CAD build for the part. Positions are in the model's coordinates, mm. Face numbers are marked on the shaded views. A direction names the side the tool comes from. Round coordinates to 2 decimals unless told otherwise and drop trailing zeros. Loops run counter-clockwise (first coordinate to the right, second up) from the corner with the lowest first, then second, coordinate; pieces in that order, holes last. Notation, with made-up numbers: M 25,63 L 84,63 A13 ccw 84,72 Z; hole C 56,32 d2. An arc over 180 degrees is marked long. Use a Markdown table: item, result. Add a question column.
(1) Band-saw the part on B-B, the plane z = 7.75. Give the number of separate pieces and of enclosed holes in the cut face, and give its area (3 significant figures).
(2) Wall check: L1, parallel to Z at x = 12.5, y = -11.5. Give the ranges that are in metal, low to high.
(3) Which spindle directions (+Z, -Z, +X, -X, +Y, -Y) get a long thin tool onto all of the face, cutting with end or side? Do the marked faces 1, 2 and 3. Say none if no direction does.
(4) Band-saw the part on C-C, the plane y = 3. Write the cut outline in (x, z).
(5) Band-saw the part on A-A, the plane y = -16. Write the cut outline in (x, z).
(6) Flat gauge pins, fed straight in: P1, Ø5, axis at x = -7.5, z = 8.5, coming from the +Y side; P2, Ø0.5, axis at y = -15, z = 5, coming from the -X side; P3, Ø3, axis at x = -5, z = 9, coming from the -Y side. Where does each tip first touch, or does it go through?
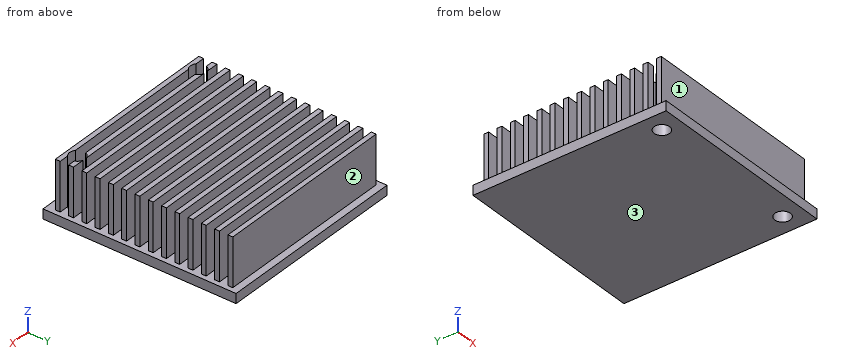
from build123d import *

# Parameters (mm, degrees)
SKETCH1_W           = 40
SKETCH1_H           = 40
BOSS_EXTRUDE1_DEPTH = 2
SKETCH2_W           = 38
SKETCH2_H           = 1
BOSS_EXTRUDE2_DEPTH = 10
SKETCH3_R           = 1.6
CUT_EXTRUDE1_DEPTH  = 13


with BuildPart() as part:
    # Sketch1 → Boss-Extrude1 (new body)
    with BuildSketch(Plane.XY):
        Rectangle(SKETCH1_W, SKETCH1_H)
    extrude(amount=BOSS_EXTRUDE1_DEPTH)

    # Sketch2 → Boss-Extrude2 (add)
    with BuildSketch(Plane.XY.offset(2)):
        with Locations((0, 15.280666702)):
            Rectangle(SKETCH2_W, SKETCH2_H)
        with Locations((0, 18.030666702)):
            Rectangle(SKETCH2_W, SKETCH2_H)
        with Locations((0, 12.530666702)):
            Rectangle(SKETCH2_W, SKETCH2_H)
        with Locations((0, 9.780666702)):
            Rectangle(SKETCH2_W, SKETCH2_H)
        with Locations((0, 7.030666702)):
            Rectangle(SKETCH2_W, SKETCH2_H)
        with Locations((0, 4.280666702)):
            Rectangle(SKETCH2_W, SKETCH2_H)
        with Locations((0, 1.530666702)):
            Rectangle(SKETCH2_W, SKETCH2_H)
        with Locations((0, -1.219333298)):
            Rectangle(SKETCH2_W, SKETCH2_H)
        with Locations((0, -3.969333298)):
            Rectangle(SKETCH2_W, SKETCH2_H)
        with Locations((0, -6.719333298)):
            Rectangle(SKETCH2_W, SKETCH2_H)
        with Locations((0, -9.469333298)):
            Rectangle(SKETCH2_W, SKETCH2_H)
        with Locations((0, -12.219333298)):
            Rectangle(SKETCH2_W, SKETCH2_H)
        with Locations((0, -14.969333298)):
            Rectangle(SKETCH2_W, SKETCH2_H)
        with Locations((0, -17.719333298)):
            Rectangle(SKETCH2_W, SKETCH2_H)
    extrude(amount=BOSS_EXTRUDE2_DEPTH)

    # Sketch3 → Cut-Extrude1 (cut, through all)
    with BuildSketch(Plane(origin=(0, 0, 0), x_dir=(-1, 0, 0), z_dir=(0, 0, -1))):
        with Locations((16, -16)):
            Circle(SKETCH3_R)
        with Locations((-16, -16)):
            Circle(SKETCH3_R)
    extrude(amount=-CUT_EXTRUDE1_DEPTH, mode=Mode.SUBTRACT)


solid = part.part
Return value:
| question | item | result |
|---|---|---|
| 1 | separate pieces | 16 |
| 1 | enclosed holes | 0 |
| 1 | area | 526 mm^2 |
| 2 | L1 | 0 to 2 |
| 3 | face 1 | +Z, +X, -X, -Y |
| 3 | face 2 | +Z, +X, -X, +Y |
| 3 | face 3 | -Z, +X, -X, +Y, -Y |
| 4 | outline | M -20,0 L 20,0 L 20,2 L -20,2 Z |
| 5 | outline | M -20,0 L -17.6,0 L -17.6,2 L -20,2 Z; M -14.4,0 L 14.4,0 L 14.4,2 L -14.4,2 Z; M 17.6,0 L 20,0 L 20,2 L 17.6,2 Z |
| 6 | P1 | y = 18.53 |
| 6 | P2 | x = -19 |
| 6 | P3 | y = -18.22 |
